Design review of the part built by this model. Coordinates are the model's own, in mm. Face numbers are marked on the shaded views. A direction names the side the tool comes from. Give positions to 0.01 mm unless a question says otherwise; leave off trailing zeros. Order: outer loops, then holes, each group sorted by start corner. A loop starts at its lowest first (then second) coordinate and runs counter-clockwise, first axis right, second up.
```python
from build123d import *

# Parameters (mm, degrees)
EXTRUDE_1_DEPTH      = 58
EXTRUDE_2_DEPTH      = 20
CUT_EXTRUDE_1_DEPTH  = 8
EXTRUDE_3_DEPTH      = 15
EXTRUDE_3_DEPTH_BACK = 15


with BuildPart() as part:
    # Эскиз1 → Бобышка-Вытянуть1 (new body)
    with BuildSketch(Plane.XY):
        Polygon((-15, 20), (-35, -20), (35, -20), (35, 20), align=None)
    extrude(amount=EXTRUDE_1_DEPTH)

    # Эскиз2 → Бобышка-Вытянуть2 (add)
    with BuildSketch(Plane(origin=(0, 20, 0), x_dir=(1, 0, 0), z_dir=(0, 1, 0))):
        with BuildLine():
            Line((29, -29), (10, -29))
            Line((10, -29), (10, -48))
            ThreePointArc((10, -48), (23.435028843, -42.435028843), (29, -29))
        make_face()
        with BuildLine():
            ThreePointArc((29, -29), (10, -10), (-9, -29))
            Line((-9, -29), (10, -29))
            Line((10, -29), (29, -29))
        make_face()
    extrude(amount=EXTRUDE_2_DEPTH)

    # Эскиз3 → Вырез-Вытянуть1 (cut)
    with BuildSketch(Plane.XY.offset(58)):
        Polygon((22, -7), (22, 7), (-6.965558146, 7), (-13.965558146, -7), align=None)
    extrude(amount=-CUT_EXTRUDE_1_DEPTH, mode=Mode.SUBTRACT)

    # Эскиз4 → Бобышка-Вытянуть3 (add, two sides: drawn at the far end of the back side and taken through both)
    with BuildSketch(Plane.XY.offset(29).offset(-EXTRUDE_3_DEPTH_BACK)):
        Polygon((-31, -12), (-31, 14), (-18, 14), align=None)
    extrude(amount=EXTRUDE_3_DEPTH + EXTRUDE_3_DEPTH_BACK)


solid = part.part
```
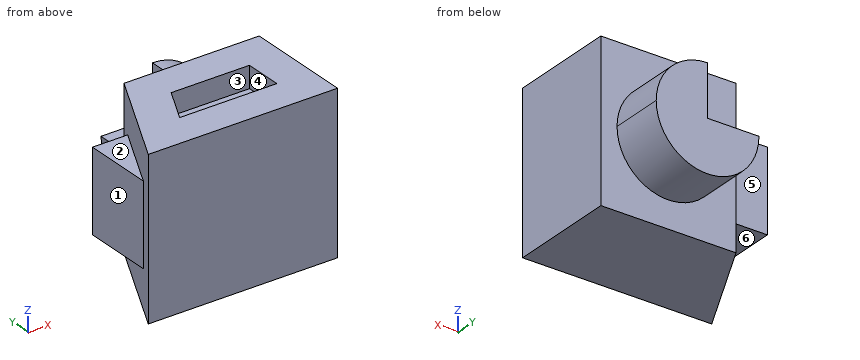
1. Take a section at C-C (x = 15.5). State the section outline as (y, z) points.
Recorded:
outline: (-20, 0) - (20, 0) - (20, 10.81) - (40, 10.81) - (40, 47.19) - (20, 47.19) - (20, 58) - (7, 58) - (7, 50) - (-7, 50) - (-7, 58) - (-20, 58) - close
2. For pin 1 (7 mm diameter, centred on x = 11, y = 0, fed in from +Z); pin 2 (13 mm diameter, centred on y = -1.5, z = 24, fed in from -X); pin 3 (4 mm diameter, centred on y = 1, z = 53, fed in from -X), all flat-tipped, find the tip position at first contact; note any pin that passes through.
Recorded:
pin 1: stops at z = 50
pin 2: stops at x = -31
pin 3: stops at x = -25.5
3. Machinability: for the marked faces 4, 5 and 6, which of the approach directions +Z, -Z, +X, -X, +Y, -Y give a long, thin tool a straight path to every point of the face, cutting with its end or side? Answer none if there is none.
Recorded:
face 4: +Z
face 5: +Z, -Z, -X, +Y
face 6: -Z, -X, +Y
4. Take a section at D-D (x = 0.5). State the section outline as (y, z) points.
Recorded:
outline: (-20, 0) - (20, 0) - (20, 12.55) - (40, 12.55) - (40, 29) - (20, 29) - (20, 58) - (7, 58) - (7, 50) - (-7, 50) - (-7, 58) - (-20, 58) - close
5. For line 1 along Y through (x, z) = (10.5, 51); line 2 along Y through (x, z) = (-9.5, 16); line 3 along Z through (x, y) = (13.5, -5), list the stretches that pass through material, from the lowest coordinate up.
Recorded:
line 1: y = -20 to -7, 7 to 20
line 2: y = -20 to 20
line 3: z = 0 to 50
6. Take a section at A-A (y = 10.5). State the section outline as (x, z) points, then the cut area to 3 significant figures.
Recorded:
outline: (-31, 14) - (-19.75, 14) - (-19.75, 0) - (35, 0) - (35, 58) - (-19.75, 58) - (-19.75, 44) - (-31, 44) - close
area: 3,510 mm2
7. Draft analysis for pull direction X (two halves, no side actions). For the marked faces 1, 2 and 3, state which applies: pulls with the +X half, pulls with the -X half, needs draft (parallel to the pull), parting line crosses it, or undercut.
Recorded:
face 1: pulls with the -X half
face 2: needs draft
face 3: undercut
8. Take a section at B-B (x = 27.5). State the section outline as (y, z) points, then the cut area to 3 significant figures.
Recorded:
outline: (-20, 0) - (20, 0) - (20, 21.6) - (40, 21.6) - (40, 36.4) - (20, 36.4) - (20, 58) - (-20, 58) - close
area: 2,620 mm2
